Can you work these out from the model? Positions are in its coordinate system, mm. Face numbers are marked on the shaded views. A direction names the side the tool comes from. Coordinates: 2 decimals unless noted, no trailing zeros. Order: outer loops, then holes, each group sorted by start corner. A loop starts at its lowest first (then second) coordinate and runs counter-clockwise, first axis right, second up. Notation, with made-up numbers: (43.25, 9.25) -> (97.25, 9.25) arc R27 cw to (97.25, 44.25) -> close; hole circle Ø1 at (89, 0.5). An arc over 180 degrees is marked (long way). Answer as CSV lines item,"result".
from build123d import *

# Parameters (mm, degrees)
SKETCH_1_W                     = 31
SKETCH_1_H                     = 40
SKETCH_1_R                     = 1.6
EXTRUDE_1_DEPTH                = 5
SKETCH_2_W                     = 31
SKETCH_2_H                     = 9.8
EXTRUDE_3_DEPTH                = 8
SKETCH_13_R                    = 1
CUT_EXTRUDE_7_DEPTH            = 5
EXTRUDE_START                  = 1
SKETCH_14_R                    = 3
SKETCH_14_R_2                  = 1
EXTRUDE_8_DEPTH                = 1
HOLE_WIZARD_M3_3_D             = 2.5
HOLE_WIZARD_M3_3_DEPTH         = 6.5
HOLE_WIZARD_M3_3_TIP           = 0.751075774
SKETCH_18_W                    = 31
SKETCH_18_H                    = 3
EXTRUDE_9_DEPTH                = 10
SKETCH_29_W                    = 31
SKETCH_29_H                    = 6.8
EXTRUDE_11_DEPTH               = 2
SKETCH_20_R                    = 1
CUT_EXTRUDE_9_DEPTH            = 9
HOLE_START                     = -9
HOLE_WIZARD_M3_1_OUTLINE_R     = 1.25
HOLE_WIZARD_M3_1_OUTLINE_R_2   = 1
HOLE_WIZARD_M3_1_DEPTH         = 9
HOLE_WIZARD_M3_1_3_D           = 3.2
HOLE_WIZARD_M3_1_3_CBORE_D     = 6
HOLE_WIZARD_M3_1_3_CBORE_DEPTH = 3.1
HOLE_START_2                   = -40
HOLE_WIZARD_M3_2_OUTLINE_R     = 1.25
HOLE_WIZARD_M3_2_OUTLINE_R_2   = 1
HOLE_WIZARD_M3_2_DEPTH         = 9
FILLET_2_R                     = 1
SKETCH_30_W                    = 31
SKETCH_30_H                    = 7
CUT_EXTRUDE_10_DEPTH           = 4


# Read off the part's stored shape, not the designer's step: M3 螺纹孔1, M3 螺纹孔2
with BuildPart() as part:
    # 草图1 → 凸台-拉伸1 (new body)
    with BuildSketch(Plane(origin=(0, 0, 0), x_dir=(1, 0, 0), z_dir=(0, 1, 0))):
        with Locations((15.5, 20)):
            Rectangle(SKETCH_1_W, SKETCH_1_H)
        with Locations(Location((20.5, 27.5, 0), (0, 0, 270))):
            Circle(SKETCH_1_R, mode=Mode.SUBTRACT)
        with Locations(Location((10.5, 27.5, 0), (0, 0, 270))):
            Circle(SKETCH_1_R, mode=Mode.SUBTRACT)
        with Locations(Location((10.5, 12.5, 0), (0, 0, 90))):
            Circle(SKETCH_1_R, mode=Mode.SUBTRACT)
        with Locations(Location((20.5, 12.5, 0), (0, 0, 90))):
            Circle(SKETCH_1_R, mode=Mode.SUBTRACT)
    extrude(amount=EXTRUDE_1_DEPTH)

    # 草图2 → 凸台-拉伸3 (add)
    with BuildSketch(Plane(origin=(0, 0, 0), x_dir=(1, 0, 0), z_dir=(0, 1, 0))):
        with Locations((15.5, 35.1)):
            Rectangle(SKETCH_2_W, SKETCH_2_H)
    extrude(amount=-EXTRUDE_3_DEPTH)

    # 草图13 → 切除-拉伸7 (cut)
    with BuildSketch(Plane.XZ.offset(8)):
        with Locations(Location((15.5, -35.1, 0), (0, 0, 270))):
            Circle(SKETCH_13_R)
    extrude(amount=-CUT_EXTRUDE_7_DEPTH, mode=Mode.SUBTRACT)

    # 草图14 → 凸台-拉伸8 (add)
    with BuildSketch(Plane.XZ.offset(8).offset(EXTRUDE_START)):
        with Locations(Location((15.5, -35.1, 0), (0, 0, 270))):
            Circle(SKETCH_14_R)
        with Locations(Location((15.5, -35.1, 0), (0, 0, 270))):
            Circle(SKETCH_14_R_2, mode=Mode.SUBTRACT)
    extrude(amount=-EXTRUDE_8_DEPTH)

    # M3 螺纹孔3
    with Locations(Plane(origin=(0, -9, 0), x_dir=(-1, 0, 0), z_dir=(0, -1, 0))):
        with Locations((-15.5, 35.1)):
            Hole(HOLE_WIZARD_M3_3_D / 2, depth=HOLE_WIZARD_M3_3_DEPTH)
            with Locations((0, 0, -(HOLE_WIZARD_M3_3_DEPTH + HOLE_WIZARD_M3_3_TIP / 2))):  # 118° drill point
                Cone(0, HOLE_WIZARD_M3_3_D / 2, HOLE_WIZARD_M3_3_TIP, mode=Mode.SUBTRACT)

    # 草图18 → 凸台-拉伸9 (add)
    with BuildSketch(Plane(origin=(0, 5, 0), x_dir=(1, 0, 0), z_dir=(0, 1, 0))):
        with Locations((15.5, 8.3)):
            Rectangle(SKETCH_18_W, SKETCH_18_H)
    extrude(amount=-EXTRUDE_9_DEPTH)

    # 草图29 → 凸台-拉伸11 (add)
    with BuildSketch(Plane.XZ):
        with Locations((15.5, -3.4)):
            Rectangle(SKETCH_29_W, SKETCH_29_H)
    extrude(amount=EXTRUDE_11_DEPTH)

    # 草图20 → 切除-拉伸9 (cut)
    with BuildSketch(Plane.XY):
        with Locations((7.5, 2)):
            Circle(SKETCH_20_R)
        with Locations(Location((23.5, 2, 0), (0, 0, 180))):
            Circle(SKETCH_20_R)
    cut_extrude_9 = extrude(amount=-CUT_EXTRUDE_9_DEPTH, mode=Mode.SUBTRACT)

    # Hole Wizard M3 _1 outline → Hole Wizard M3 _1 (cut)
    with BuildSketch(Plane.XY.offset(HOLE_START)):
        with Locations((23.5, 2)):
            Circle(HOLE_WIZARD_M3_1_OUTLINE_R)
        with Locations((23.5, 2)):
            Circle(HOLE_WIZARD_M3_1_OUTLINE_R_2, mode=Mode.SUBTRACT)
    extrude(amount=HOLE_WIZARD_M3_1_DEPTH, mode=Mode.SUBTRACT)

    # Hole Wizard M3 _1 2 outline → Hole Wizard M3 _1 2 (revolve, cut)
    with BuildSketch(Plane(origin=(7.5, 2, 0), x_dir=(1, 0, 0), z_dir=(0, -1, 0))):
        Polygon((0, -9), (0, -9.751075774), (1.25, -9), (1.25, 0), (1, 0), (1, -9), align=None)
    revolve(axis=Axis((7.5, 2, 0), (0, 0, 1)), mode=Mode.SUBTRACT)

    # 镜向1: 切除-拉伸9 across plane
    add(cut_extrude_9.mirror(Plane.XY.offset(-20)), mode=Mode.SUBTRACT)

    # Hole Wizard M3 _1 3 (through all)
    with Locations(Plane(origin=(0, 5, 0), x_dir=(1, 0, 0), z_dir=(0, 1, 0))):
        with Locations((10.5, 27.5), (10.5, 12.5), (20.5, 12.5), (20.5, 27.5)):
            CounterBoreHole(HOLE_WIZARD_M3_1_3_D / 2, HOLE_WIZARD_M3_1_3_CBORE_D / 2, HOLE_WIZARD_M3_1_3_CBORE_DEPTH)

    # M3 螺纹孔2 outline → M3 螺纹孔2 (cut)
    with BuildSketch(Plane.XY.offset(HOLE_START_2)):
        with Locations((7.5, 2)):
            Circle(HOLE_WIZARD_M3_2_OUTLINE_R)
        with Locations((7.5, 2)):
            Circle(HOLE_WIZARD_M3_2_OUTLINE_R_2, mode=Mode.SUBTRACT)
    extrude(amount=HOLE_WIZARD_M3_2_DEPTH, mode=Mode.SUBTRACT)

    # Hole Wizard M3 _2 2 outline → Hole Wizard M3 _2 2 (revolve, cut)
    with BuildSketch(Plane(origin=(23.5, 2, 0), x_dir=(1, 0, 0), z_dir=(0, -1, 0))):
        Polygon((1.25, -31), (0, -30.248924226), (0, -31), (1, -31), (1, -40), (1.25, -40), align=None)
    revolve(axis=Axis((23.5, 2, 0), (0, 0, 1)), mode=Mode.SUBTRACT)

    # 圆角2
    fillet_2_edges = [part.edges().sort_by_distance(p)[0] for p in [
        (15.5, -2, -6.8),
    ]]
    fillet(fillet_2_edges, radius=FILLET_2_R)

    # 草图30 → 切除-拉伸10 (cut)
    with BuildSketch(Plane.XY):
        with Locations((15.5, 1.5)):
            Rectangle(SKETCH_30_W, SKETCH_30_H)
    cut_extrude_10 = extrude(amount=-CUT_EXTRUDE_10_DEPTH, mode=Mode.SUBTRACT)

    # 镜向3: 切除-拉伸10 across plane
    add(cut_extrude_10.mirror(Plane.XY.offset(-20)), mode=Mode.SUBTRACT)


solid = part.part
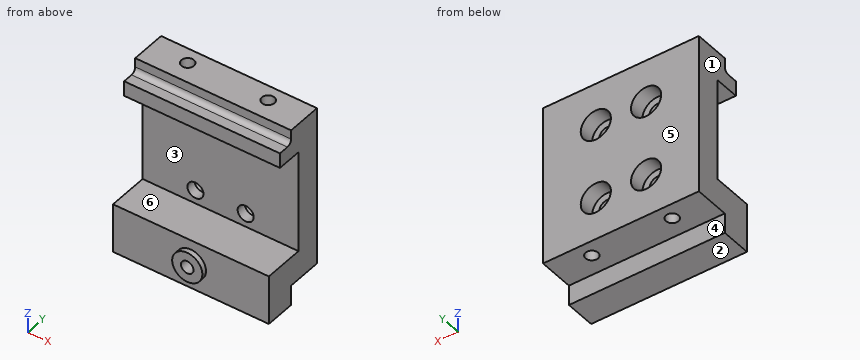
Q1. Which directions (+Z, -Z, +X, -X, +Y, -Y) give clear straight access to the entire face, cutting with the end or side of a thin tool? Please do the marked faces 4, 5 and 6.
Solution:
face 4,"-Z, +X, -X, +Y"
face 5,"+Z, -Z, +X, -X, +Y"
face 6,"+X, -X, -Y"
Q2. Imagine slicing it at C-C (z = -8). List the corners of the cut face in (x, y) for me, and give its area (3 significant figures).
Solution:
outline,"(0, -5) -> (31, -5) -> (31, 5) -> (0, 5) -> close; hole circle Ø2.5 at (7.5, 2); hole circle Ø2.5 at (23.5, 2)"
area,"300 mm2"
Q3. Imagine slicing it at D-D (y = -6). List the corners of the cut face in (x, z) for me, and give its area (3 significant figures).
Solution:
outline,"(0, -40) -> (31, -40) -> (31, -30.2) -> (0, -30.2) -> close; hole circle Ø2.5 at (15.5, -35.1)"
area,"299 mm2"
Q4. We'd pull the mould along Z, two halves only. Please class the marked faces 1, 2 and 3: pulls with the +Z half, pulls with the -Z half, needs draft (parallel to the pull), parting line crosses it, or undercut.
Solution:
face 1,"needs draft"
face 2,"pulls with the -Z half"
face 3,"undercut"
Q5. Imagine slicing it at B-B (x = 10.5). Give the number of separate pieces and of enclosed holes in the cut face, and give its area (3 significant figures).
Solution:
separate pieces,"3"
enclosed holes,"0"
area,"202 mm2"
Q6. If I drill on line 1 (X direction, y = 4, z = -27.5); line 2 (X direction, y = 1.3, z = -27.5); line 3 (Z direction, x = 2.5, y = -0.75), over which ranges is the centre line in solid material (lowest first)?
Solution:
line 1,"0 to 7.5, 13.5 to 17.5, 23.5 to 31"
line 2,"0 to 8.9, 12.1 to 18.9, 22.1 to 31"
line 3,"-36 to -30.2, -9.8 to -4"
Q7. For P1, Ø3, axis at x = 11.5, z = -12.5, coming from the +Y side; P2, Ø7.5, axis at x = 11, y = 0, coming from the -Z side; P3, Ø1.8, axis at x = 21, z = -27.5, coming from the +Y side; P4, Ø5.5, axis at x = 10.5, z = -27.5, coming from the -Y side, each with a flat end and sliding along its axis, tell me the tip position at first contact or that it passes through.
Solution:
P1,"y = 1.9"
P2,"z = -40"
P3,"through"
P4,"y = -8"
Q8. Imagine slicing it at A-A (z = -12.5). List the corners of the cut face in (x, y) for me.
Solution:
outline,"(0, 0) -> (8.9, 0) -> (8.9, 1.9) -> (7.5, 1.9) -> (7.5, 5) -> (0, 5) -> close; (12.1, 0) -> (18.9, 0) -> (18.9, 1.9) -> (17.5, 1.9) -> (17.5, 5) -> (13.5, 5) -> (13.5, 1.9) -> (12.1, 1.9) -> close; (22.1, 0) -> (31, 0) -> (31, 5) -> (23.5, 5) -> (23.5, 1.9) -> (22.1, 1.9) -> close"
